Here's the drawing with two shaded views (mm, measured from the low corner). I have some questions. A direction names the side the tool comes from. Give positions to 0.01 mm unless a question says otherwise; leave off trailing zeros. Order: outer loops, then holes, each group sorted by start corner. A loop starts at its lowest first (then second) coordinate and runs counter-clockwise, first axis right, second up. Notation, with made-up numbers: M 35,65 L 47,65 A23 cw 47,96 Z; hole C -3,10.5 d7. An arc over 180 degrees is marked long. One line per question, with ' | ' between items. Start each with the question number.
1) Please list where these lines run through material, in increasing order: line 1 along Z through (x, y) = (224, 23) (1 decimal); line 2 along X through (y, z) = (31, 109.5) (3 decimals); line 3 along Z through (x, y) = (11.5, 32). Write a range as [from, to].
2) If we section it at B-B, the plane z = 30: Please give me the cut outline in (x, y) (3 decimals), plus the area to 3 significant figures.
3) Thinking about a two-plate mould opening in X: for the marked faces 3, 4 and 5, which applies, +X half, -X half, draft (parallel to the pull), parting line (faces both ways), or undercut?
4) If we section it at A-A, the plane y = 23: Please give me the cut outline in (x, z) (1 decimal).
5) If we section it at C-C, the plane x = 204.5: Please give me the cut outline in (y, z), plus the area to 3 significant figures.
6) I'm going to push a flat-ended pin straight in: pin 1 Ø1.5 at (x, z) = (198.5, 180) entering from +Y. Where does the tip first touch, or does it pass through?
7) For the marked faces 1 and 2, which set-ups out of +Z, -Z, +X, -X, +Y, -Y let a thin tool reach every point of the face, with its end or its side?
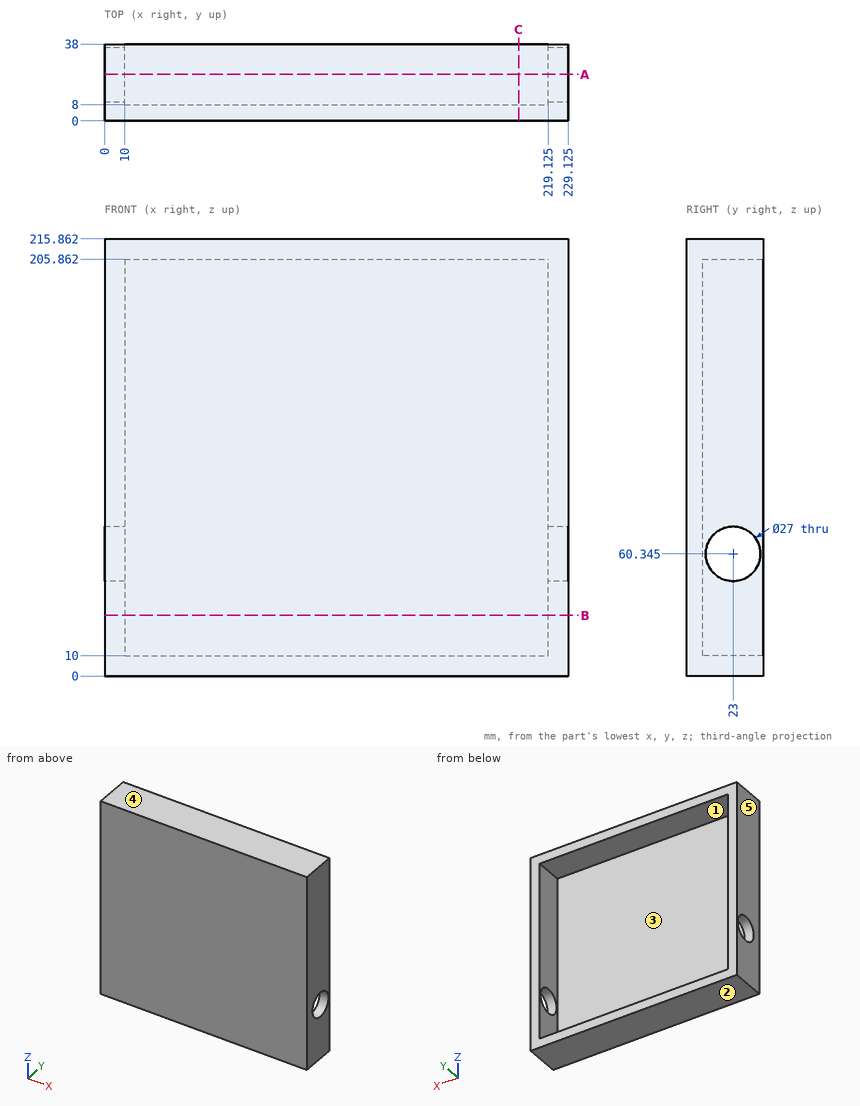
Results found:
1) line 1: z = [0, 46.8], [73.8, 215.9] | line 2: x = [0, 10], [219.125, 229.125] | line 3: z = [0, 10], [205.86, 215.86]
2) outline: M 0,0 L 229.125,0 L 229.125,38 L 219.125,38 L 219.125,8 L 10,8 L 10,38 L 0,38 Z | area: 2,430 mm²
3) face 3: undercut | face 4: draft | face 5: -X half
4) outline: M 0,0 L 229.1,0 L 229.1,46.8 L 219.1,46.8 L 219.1,10 L 10,10 L 10,46.8 L 0,46.8 Z; M 0,73.8 L 10,73.8 L 10,205.9 L 219.1,205.9 L 219.1,73.8 L 229.1,73.8 L 229.1,215.9 L 0,215.9 Z
5) outline: M 0,0 L 38,0 L 38,10 L 8,10 L 8,205.86 L 38,205.86 L 38,215.86 L 0,215.86 Z | area: 2,330 mm²
6) pin 1: stops at y = 8
7) face 1: +Y | face 2: -Z, +X, -X, +Y, -Y
